CAD build for the part. Positions are in the model's coordinates, mm. Face numbers are marked on the shaded views. Round coordinates to 2 decimals unless told otherwise and drop trailing zeros. Order: outer loops, then holes, each group sorted by start corner. A loop starts at its lowest first (then second) coordinate and runs counter-clockwise, first axis right, second up. Notation, with made-up numbers: M 27,54.25 L 73,54.25 A26 ccw 73,79.25 Z; hole C 42,10 d6. An arc over 180 degrees is marked long. Put each result on its own line as item: value.
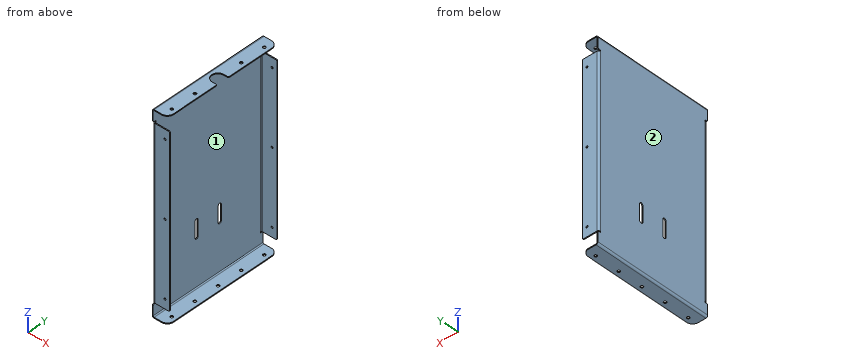
```python
from build123d import *

# Parameters (mm, degrees)
BRIDA_BASE1_DEPTH           = 95
CROQUIS4_W                  = 274
CROQUIS4_H                  = 4.5
CORTAR_EXTRUIR1_DEPTH       = 10
BRIDA_DE_ARISTA1_DEPTH      = 270
BRIDA_DE_ARISTA1_BEND_DEPTH = 270
MATRIZL1_COUNT              = 3
MATRIZL1_PITCH              = 40
MATRIZL1_COL_COUNT          = 3
MATRIZL1_COL_PITCH          = 40
REDONDEO1_R                 = 10
TALADRO_ROSCADO_M41_D       = 3.3
MATRIZL2_COUNT              = 2
MATRIZL2_PITCH              = 120
MATRIZL2_COL_COUNT          = 2
MATRIZL2_COL_PITCH          = 120
CORTAR_EXTRUIR3_DEPTH       = 10
REDONDEO2_R                 = 2
CORTAR_EXTRUIR4_DEPTH       = 10


# Sheet-metal steps are written as plain solids
with BuildPart() as part:
    # Croquis1 → Brida base1 (new, symmetric)
    with BuildSketch(Plane(origin=(0, 0, 0), x_dir=(1, 0, 0), z_dir=(0, 1, 0))):
        with BuildLine():
            Line((25, -156.65), (3, -156.65))
            ThreePointArc((3, -156.65), (0.878679656, -155.771320344), (0, -153.65))
            Line((0, -153.65), (0, 153.65))
            ThreePointArc((0, 153.65), (0.878679656, 155.771320344), (3, 156.65))
            Line((3, 156.65), (25, 156.65))
            Line((25, 156.65), (25, 155.15))
            Line((25, 155.15), (3, 155.15))
            ThreePointArc((3, 155.15), (1.939339828, 154.710660172), (1.5, 153.65))
            Line((1.5, 153.65), (1.5, -153.65))
            ThreePointArc((1.5, -153.65), (1.939339828, -154.710660172), (3, -155.15))
            Line((3, -155.15), (25, -155.15))
            Line((25, -155.15), (25, -156.65))
        make_face()
    extrude(amount=BRIDA_BASE1_DEPTH, both=True)

    # Croquis4 → Cortar-Extruir1 (cut)
    with BuildSketch(Plane.ZY):
        with Locations((0, 92.75)):
            Rectangle(CROQUIS4_W, CROQUIS4_H)
    cortar_extruir1 = extrude(amount=-CORTAR_EXTRUIR1_DEPTH, mode=Mode.SUBTRACT)

    # Simetría3: Cortar-Extruir1 across plane
    add(cortar_extruir1.mirror(Plane.ZX), mode=Mode.SUBTRACT)

    # Brida de arista1 section (across the edge) → Brida de arista1 (add)
    with BuildSketch(Plane(origin=(1.5, 92, -135), x_dir=(0, -1, 0), z_dir=(0, 0, 1))):
        with BuildLine():
            Line((-1.5, 1.5), (-1.5, 25))
            Line((-1.5, 25), (0, 25))
            Line((0, 25), (0, 1.5))
            ThreePointArc((0, 1.5), (0.439339828, 0.439339828), (1.5, 0))
            Line((1.5, 0), (1.5, -1.5))
            ThreePointArc((1.5, -1.5), (-0.621320344, -0.621320344), (-1.5, 1.5))
        make_face()
    extrude(amount=BRIDA_DE_ARISTA1_DEPTH)

    # Brida de arista1 section 2 (across the edge) → Brida de arista1 bend (add)
    with BuildSketch(Plane(origin=(1.5, -92, 135), x_dir=(0, 1, 0), z_dir=(0, 0, -1))):
        with BuildLine():
            Line((-1.5, 1.5), (-1.5, 25))
            Line((-1.5, 25), (0, 25))
            Line((0, 25), (0, 1.5))
            ThreePointArc((0, 1.5), (0.439339828, 0.439339828), (1.5, 0))
            Line((1.5, 0), (1.5, -1.5))
            ThreePointArc((1.5, -1.5), (-0.621320344, -0.621320344), (-1.5, 1.5))
        make_face()
    extrude(amount=BRIDA_DE_ARISTA1_BEND_DEPTH)

    # Croquis11 → Taladro de margen para M41 (revolve, cut)
    with BuildSketch(Plane(origin=(17.5, 0, -156.65), x_dir=(0, 1, 0), z_dir=(1, 0, 0))):
        Polygon((0, 0), (0, 501.351936393), (2.25, 500), (2.25, 0), align=None)
    taladro_de_margen_para_m41 = revolve(axis=Axis((17.5, 0, -163), (0, 0, 1)), mode=Mode.SUBTRACT)

    # MatrizL1: Taladro de margen para M41 ×3
    with Locations(*[(0, -i * MATRIZL1_PITCH, 0) for i in range(1, MATRIZL1_COUNT)]):
        add(taladro_de_margen_para_m41, mode=Mode.SUBTRACT)

    # MatrizL1 col: Taladro de margen para M41 ×3
    with Locations(*[(0, i * MATRIZL1_COL_PITCH, 0) for i in range(1, MATRIZL1_COL_COUNT)]):
        add(taladro_de_margen_para_m41, mode=Mode.SUBTRACT)

    # Redondeo1
    redondeo1_edges = [part.edges().sort_by_distance(p)[0] for p in [
        (25, -95, 155.9),
        (25, -95, -155.9),
        (25, 95, 155.9),
        (25, 95, -155.9),
    ]]
    fillet(redondeo1_edges, radius=REDONDEO1_R)

    # Taladro roscado M41 (through all)
    with Locations(Plane(origin=(0, 93.5, 0), x_dir=(1, 0, 0), z_dir=(0, 1, 0))):
        with Locations((19, 0)):
            taladro_roscado_m41 = Hole(TALADRO_ROSCADO_M41_D / 2)

    # MatrizL2: Taladro roscado M41 ×2
    with Locations(*[(0, 0, i * MATRIZL2_PITCH) for i in range(1, MATRIZL2_COUNT)]):
        add(taladro_roscado_m41, mode=Mode.SUBTRACT)

    # MatrizL2 col: Taladro roscado M41 ×2
    with Locations(*[(0, 0, -i * MATRIZL2_COL_PITCH) for i in range(1, MATRIZL2_COL_COUNT)]):
        add(taladro_roscado_m41, mode=Mode.SUBTRACT)

    # Croquis20 → Cortar-Extruir3 (cut)
    with BuildSketch(Plane(origin=(0, 0, 155.15), x_dir=(-1, 0, 0), z_dir=(0, 0, -1))):
        with BuildLine():
            Line((-17.5, -10), (-25, -10))
            ThreePointArc((-25, -10), (-35, 0), (-25, 10))
            Line((-25, 10), (-17.5, 10))
            ThreePointArc((-17.5, 10), (-7.5, 0), (-17.5, -10))
        make_face()
    extrude(amount=-CORTAR_EXTRUIR3_DEPTH, mode=Mode.SUBTRACT)

    # Redondeo2
    redondeo2_edges = [part.edges().sort_by_distance(p)[0] for p in [
        (26.5, -92.75, 135),
        (26.5, -92.75, -135),
        (25, -10, 155.9),
        (25, 10, 155.9),
        (0.75, 95, -137),
        (0.75, 95, 137),
        (0.75, -95, -137),
        (0.75, -95, 137),
        (26.5, 92.75, -135),
        (26.5, 92.75, 135),
    ]]
    fillet(redondeo2_edges, radius=REDONDEO2_R)

    # Croquis21 → Cortar-Extruir4 (cut)
    with BuildSketch(Plane.ZY):
        with BuildLine():
            Line((-79.15, -17.25), (-54.15, -17.25))
            ThreePointArc((-54.15, -17.25), (-51.4, -20), (-54.15, -22.75))
            Line((-54.15, -22.75), (-79.15, -22.75))
            ThreePointArc((-79.15, -22.75), (-81.9, -20), (-79.15, -17.25))
        make_face()
        with BuildLine():
            Line((-79.15, 22.75), (-54.15, 22.75))
            ThreePointArc((-54.15, 22.75), (-51.4, 20), (-54.15, 17.25))
            Line((-54.15, 17.25), (-79.15, 17.25))
            ThreePointArc((-79.15, 17.25), (-81.9, 20), (-79.15, 22.75))
        make_face()
    extrude(amount=-CORTAR_EXTRUIR4_DEPTH, mode=Mode.SUBTRACT)


solid = part.part
```
Item 1: Band-saw the part on B-B on y = 60. Give the cut face in (x, z).
Answers below:
outline: M 0,-153.65 A3 ccw 3,-156.65 L 25,-156.65 L 25,-155.15 L 3,-155.15 A1.5 cw 1.5,-153.65 L 1.5,153.65 A1.5 cw 3,155.15 L 25,155.15 L 25,156.65 L 3,156.65 A3 ccw 0,153.65 Z
Item 2: Pin check, flat tips, straight feed: P1, Ø1.2, axis at x = 0.5, z = -68, coming from the +Y side; P2, Ø7, axis at x = 14, z = -16, coming from the -Y side; P3, Ø3, axis at y = 48, z = -109.5, coming from the +X side. Stop position of each tip, or through.
Answers below:
P1: y = 92.82
P2: y = -93.5
P3: x = 1.5
Item 3: Band-saw the part on C-C on x = 12. Give the cut face in (y, z), and give its area (3 significant figures).
Answers below:
outline: M -95,-156.65 L 95,-156.65 L 95,-155.15 L -95,-155.15 Z; M -95,155.15 L -8.35,155.15 L -8.35,156.65 L -95,156.65 Z; M -93.5,-135 L -92,-135 L -92,135 L -93.5,135 Z; M 8.35,155.15 L 95,155.15 L 95,156.65 L 8.35,156.65 Z; M 92,-135 L 93.5,-135 L 93.5,135 L 92,135 Z
area: 1,350 mm²
Item 4: Mould opens along Y. For the marked faces 1 and 2 say: pulls with the +Y half, pulls with the -Y half, needs draft (parallel to the pull), parting line crosses it, or undercut.
Answers below:
face 1: undercut
face 2: needs draft
Item 5: Band-saw the part on D-D on z = -30. Give the cut face in (x, y), and give its area (3 significant figures).
Answers below:
outline: M 0,-90.5 A3 ccw 3,-93.5 L 26.5,-93.5 L 26.5,-92 L 3,-92 A1.5 cw 1.5,-90.5 L 1.5,90.5 A1.5 cw 3,92 L 26.5,92 L 26.5,93.5 L 3,93.5 A3 ccw 0,90.5 Z
area: 353 mm²
Item 6: Probe line 1 along Z through (x, y) = (19, -92.5); line 2 along Z through (x, y) = (20.75, 61); line 3 along Y through (x, z) = (10.25, -40). List the from-to ranges inside material, lowest first. Write a range as [from, to].
Answers below:
line 1: [-156.65, -155.15], [-135, -121.65], [-118.35, -1.65], [1.65, 118.35], [121.65, 135], [155.15, 156.65]
line 2: [-156.65, -155.15], [155.15, 156.65]
line 3: [-93.5, -92], [92, 93.5]
Item 7: Band-saw the part on A-A on z = -70. Give the cut face in (x, y).
Answers below:
outline: M 0,-90.5 A3 ccw 3,-93.5 L 26.5,-93.5 L 26.5,-92 L 3,-92 A1.5 cw 1.5,-90.5 L 1.5,-22.75 L 0,-22.75 Z; M 0,-17.25 L 1.5,-17.25 L 1.5,17.25 L 0,17.25 Z; M 0,22.75 L 1.5,22.75 L 1.5,90.5 A1.5 cw 3,92 L 26.5,92 L 26.5,93.5 L 3,93.5 A3 ccw 0,90.5 Z
